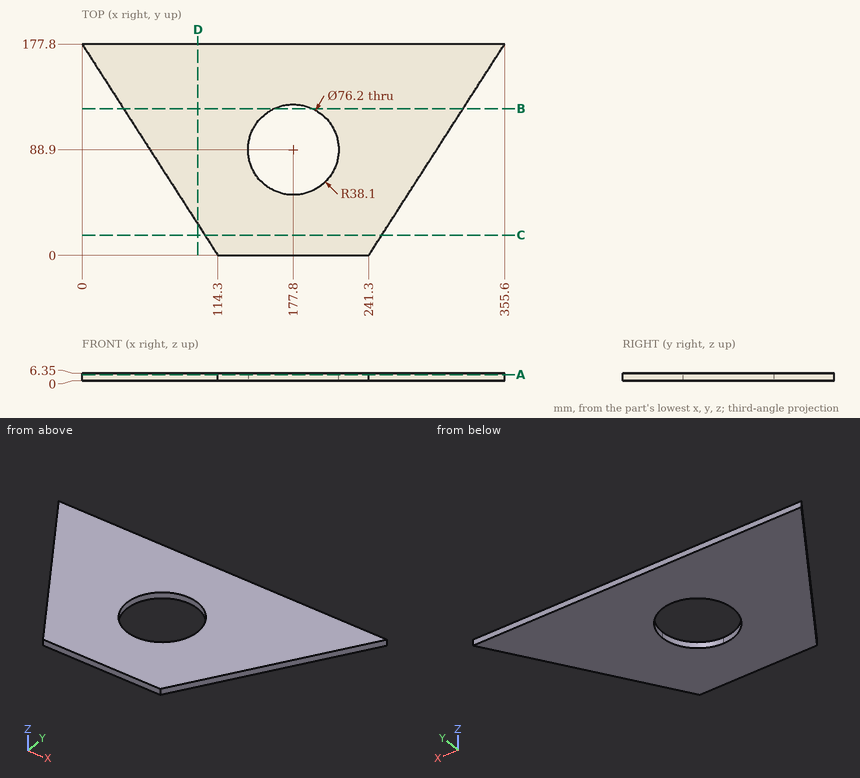
Design review of the part shown in the three views and the two pictorial views. Dimensions are in mm from the part's minimum x, y and z. Coordinates: 2 decimals unless noted, no trailing zeros. Write each loop counter-clockwise with the first axis right and the second up, starting at its lowest first coordinate (ties: lowest second). Pieces come first, ordered by that corner, then holes. Notation, with made-up numbers: (-32, 62) -> (-28, 62) arc R19 cw to (-28, 69) -> close; hole circle Ø11 at (-13.5, 17.25). An arc over 180 degrees is marked (long way). Answer in a Markdown table with one row per item.
1. We need section D-D, the plane x = 97.5. State the section outline as (y, z) points.
Answers below:
| item | result |
|---|---|
| outline | (26.13, 0) -> (177.8, 0) -> (177.8, 6.35) -> (26.13, 6.35) -> close |
2. We need section C-C, the plane y = 17. State the section outline as (x, z) points.
Answers below:
| item | result |
|---|---|
| outline | (103.37, 0) -> (252.23, 0) -> (252.23, 6.35) -> (103.37, 6.35) -> close |
3. Wall thickness on probe 1 along Y at (x, z) = (177.8, 1.75); probe 2 along Y at (x, z) = (213, 3); probe 3 along X at (y, z) = (88.9, 3.75): over which ranges is each line inside the solid? List them lowest first. Write a range as [from, to].
Answers below:
| item | result |
|---|---|
| probe 1 | y = [0, 50.8], [127, 177.8] |
| probe 2 | y = [0, 74.32], [103.48, 177.8] |
| probe 3 | x = [57.15, 139.7], [215.9, 298.45] |
4. Clearance check with flat-ended pins moving along their axes: pin 1 Ø1.5 at (y, z) = (138.5, 2.5) entering from -X; pin 2 Ø1.5 at (x, z) = (77, 1) entering from -Y. State where each tip first meets the part, or that it passes through.
Answers below:
| item | result |
|---|---|
| pin 1 | stops at x = 24.78 |
| pin 2 | stops at y = 56.86 |
5. We need section A-A, the plane z = 5.25. State the section outline as (x, y) points.
Answers below:
| item | result |
|---|---|
| outline | (0, 177.8) -> (114.3, 0) -> (241.3, 0) -> (355.6, 177.8) -> close; hole (177.8, 50.8) arc R38.1 ccw to (215.9, 88.9) arc R38.1 ccw (long way) to start |
6. We need section B-B, the plane y = 123.5. State the section outline as (x, z) points, and give its area (3 significant figures).
Answers below:
| item | result |
|---|---|
| outline | (34.91, 0) -> (161.85, 0) -> (161.85, 6.35) -> (34.91, 6.35) -> close; (193.75, 0) -> (320.69, 0) -> (320.69, 6.35) -> (193.75, 6.35) -> close |
| area | 1,610 mm^2 |
